```python
from build123d import *

# Parameters (mm, degrees)
F0_W     = 25.4
F0_H     = 50.8
F1_DEPTH = 25.4
F3_DEPTH = 12.7


with BuildPart() as f1:
    # F0 (on Front) → F1 (new body)
    with BuildSketch(Plane.XZ):
        with Locations((-13.86246, 25.4)):
            Rectangle(F0_W, F0_H)
    extrude(amount=F1_DEPTH)

    # F2 (on face) → F3 (join)
    with BuildSketch(Plane(origin=(-26.56246, 0, 0), x_dir=(0, -1, 0), z_dir=(-1, 0, 0))):
        Polygon((9.253424, -10.877157), (6.945989, 12.665603), (-18.326523, 10.123924), (-15.784844, -15.148588), align=None)
    extrude(amount=F3_DEPTH)


solid = f1.part
```
The model under review builds one solid part; all positions refer to its coordinate system, in mm. A direction names the side the tool comes from. Round coordinates to 2 decimals unless told otherwise and drop trailing zeros. Write each loop counter-clockwise with the first axis right and the second up, starting at its lowest first coordinate (ties: lowest second). Pieces come first, ordered by that corner, then holes. Notation, with made-up numbers: (-8, 69.25) - (5, 69.25) arc R34 ccw to (5, 107.25) - close; hole circle Ø7 at (61, 47.5). An arc over 180 degrees is marked (long way). Use one line per item in the form item = value.
Q1. Consider section C-C (z = 5). State the section outline as (x, y) points, and give its area (3 significant figures).
Answer key:
outline = (-39.26, -7.7) - (-26.56, -7.7) - (-26.56, -25.4) - (-1.16, -25.4) - (-1.16, 0) - (-26.56, 0) - (-26.56, 17.81) - (-39.26, 17.81) - close
area = 969 mm2
Q2. Consider section D-D (y = -11). State the section outline as (x, z) points.
Answer key:
outline = (-26.56, 0) - (-1.16, 0) - (-1.16, 50.8) - (-26.56, 50.8) - close
Q3. For line 1 (X direction, y = -18, z = 37); line 2 (Y direction, x = -5, z = 3.5); line 3 (X direction, y = 0.5, z = 0), list the stretches that pass through material, from the lowest coordinate up. Write a range as [from, to].
Answer key:
line_1 = [-26.56, -1.16]
line_2 = [-25.4, 0]
line_3 = [-39.26, -26.56]
Q4. Consider section A-A (y = -6). State the section outline as (x, z) points, and give its area (3 significant figures).
Answer key:
outline = (-39.26, -11.43) - (-26.56, -11.43) - (-26.56, 0) - (-1.16, 0) - (-1.16, 50.8) - (-26.56, 50.8) - (-26.56, 12.57) - (-39.26, 12.57) - close
area = 1,600 mm2
Q5. Insertion check: pin 1 Ø4 at (x, z) = (-8.5, 5) entering from +Y; pin 2 Ø20.5 at (x, y) = (-14, -10.5) entering from -Z; pin 3 Ø3 at (x, y) = (-34.5, 5.5) entering from -Z. Each pin has a flat end and moves straight along its axis. Give the tip position at first contact, or say it passes through.
Answer key:
pin_1 = 0
pin_2 = 0
pin_3 = -13.65
Q6. Consider section B-B (x = -27.5). State the section outline as (y, z) points.
Answer key:
outline = (-9.25, -10.88) - (15.78, -15.15) - (18.33, 10.12) - (-6.95, 12.67) - close
Q7. Tool access review of faces 1 (the flat face through (-14, 0, 26)), 2 (the flat face through (-14, -13, 0)), 3 (the flat face through (-32.824, -8.116, 0.729)): name each direction out of +Z, -Z, +X, -X, +Y, -Y from which nothing blocks a thin tool from reaching the whole face with its end or side.
Answer key:
face_1 = +Z, -Z, +X, +Y
face_2 = -Z, +X, +Y, -Y
face_3 = +Z, -X, -Y
